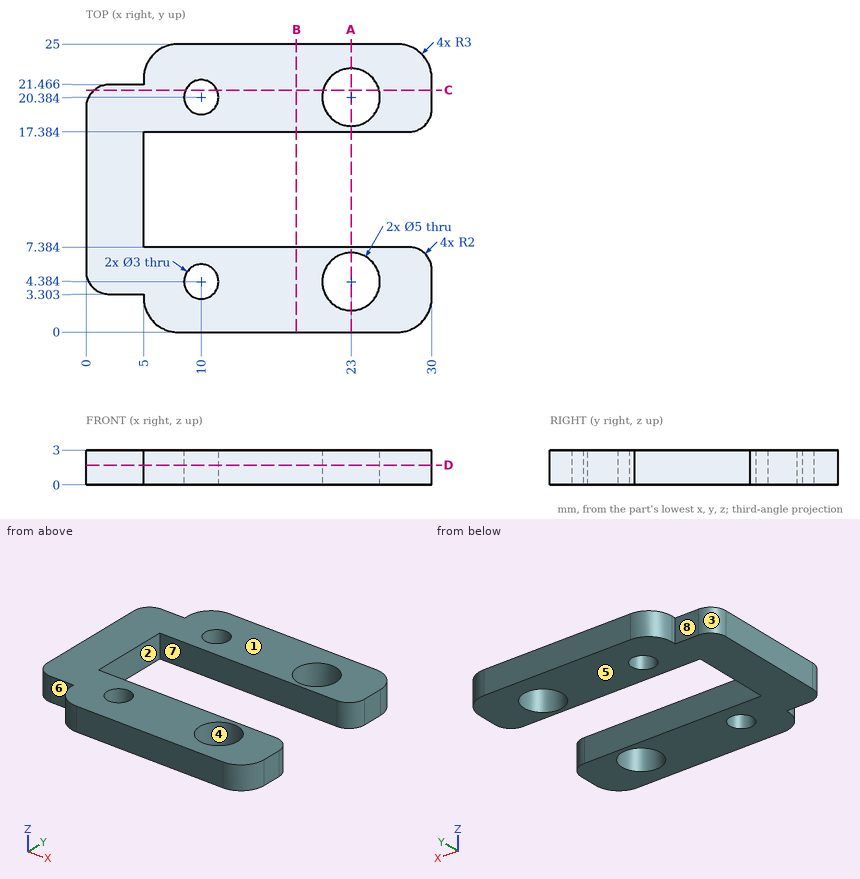
The drawing under review shows one solid part. Ordinate dimensions are in mm from its lowest x, y, z. A direction names the side the tool comes from. Coordinates: 2 decimals unless noted, no trailing zeros. Write each loop counter-clockwise with the first axis right and the second up, starting at its lowest first coordinate (ties: lowest second). Pieces come first, ordered by that corner, then holes. Notation, with made-up numbers: M 59,-6.75 L 72,-6.75 A25 ccw 72,27.25 Z; hole C -8,11 d6. An arc over 180 degrees is marked long. Answer as a JSON object with one key per item and string values.
Item 1: Draft analysis for pull direction Y (two halves, no side actions). For the marked faces 1, 2 and 3, state which applies: pulls with the +Y half, pulls with the -Y half, needs draft (parallel to the pull), parting line crosses it, or undercut.
Outcome:
{"face 1": "needs draft", "face 2": "undercut", "face 3": "pulls with the +Y half"}
Item 2: Wall thickness on probe 1 along Y at (x, z) = (23, 0.8) (1 decimal); probe 2 along Y at (x, z) = (13, 1.9) (1 decimal); probe 3 along Y at (x, z) = (10, 0.8) (1 decimal): over which ranges is each line inside the solid? List them lowest first.
Outcome:
{"probe 1": "0 to 1.9, 6.9 to 7.4, 17.4 to 17.9, 22.9 to 25", "probe 2": "0 to 7.4, 17.4 to 25", "probe 3": "0 to 2.9, 5.9 to 7.4, 17.4 to 18.9, 21.9 to 25"}
Item 3: Add section B-B, the plane x = 18.25. Give the boundary of the cut face in (y, z) (1 decimal).
Outcome:
{"outline": "M 0,0 L 7.4,0 L 7.4,3 L 0,3 Z; M 17.4,0 L 25,0 L 25,3 L 17.4,3 Z"}
Item 4: Insertion check: pin 1 Ø1.5 at (x, y) = (27, 19) entering from -Z; pin 2 Ø1.5 at (y, z) = (13, 2) entering from +X; pin 3 Ø1.5 at (x, z) = (4, 2) entering from +Y. Each pin has a flat end and moves straight along its axis. Give the tip position at first contact, or say it passes through.
Outcome:
{"pin 1": "z = 0", "pin 2": "x = 5", "pin 3": "y = 21.47"}
Item 5: Add section D-D, the plane z = 1.7. State how many separate pieces and enclosed holes the cut face has, and give its area (3 significant figures).
Outcome:
{"separate pieces": "1", "enclosed holes": "4", "area": "401 mm²"}
Item 6: Machinability: for the marked faces 4, 5, 6, 7 and 8, which of the approach directions +Z, -Z, +X, -X, +Y, -Y give a long, thin tool a straight path to every point of the face, cutting with its end or side? Answer none if there is none.
Outcome:
{"face 4": "+Z, -Z", "face 5": "-Z, +X, -X, +Y, -Y", "face 6": "+Z, -Z, -X, -Y", "face 7": "+Z, -Z, +X", "face 8": "+Z, -Z, -X, +Y"}
Item 7: Add section A-A, the plane x = 23. Give the boundary of the cut face in (y, z) (1 decimal), and give its area (3 significant figures).
Outcome:
{"outline": "M 0,0 L 1.9,0 L 1.9,3 L 0,3 Z; M 6.9,0 L 7.4,0 L 7.4,3 L 6.9,3 Z; M 17.4,0 L 17.9,0 L 17.9,3 L 17.4,3 Z; M 22.9,0 L 25,0 L 25,3 L 22.9,3 Z", "area": "15.0 mm²"}
Item 8: Add section C-C, the plane y = 21. Give the boundary of the cut face in (x, z).
Outcome:
{"outline": "M 0.72,0 L 8.63,0 L 8.63,3 L 0.72,3 Z; M 11.37,0 L 20.58,0 L 20.58,3 L 11.37,3 Z; M 25.42,0 L 30,0 L 30,3 L 25.42,3 Z"}
